Model file for the job. Use its own axes, mm. A direction names the side the tool comes from. Give positions to 0.01 mm unless a question says otherwise; leave off trailing zeros. Order: outer loops, then holes, each group sorted by start corner. A loop starts at its lowest first (then second) coordinate and runs counter-clockwise, first axis right, second up. Notation, with made-up numbers: (33, -26) -> (46, -26) arc R30 cw to (46, 7) -> close; hole circle Ø2 at (68, 55.25). An arc over 180 degrees is marked (long way). Use CSV: the item, a comma, the result in double quotes. Start each with the question number.
1. Cut at C-C on y = -6.25. List the corners of the cut face in (x, z), then the cut area to 3 significant figures.
2. Wall check: line 1 (Y direction, x = 0, z = 5.65); line 2 (X direction, y = 8, z = 11.5); line 3 (X direction, y = 1.5, z = 15.25). Give the ranges that are in metal, low to high. Write a range as from..to.
3. Cut at A-A on z = 10.5. List the corners of the cut face in (x, y), then the cut area to 3 significant figures.
4. Cut at D-D on x = 11.5. List the corners of the cut face in (y, z).
5. Drop flat-ended pins along their axis: pin 1 (2.5 mm diameter, centred on y = -7, z = 3, fed in from +X); pin 2 (1 mm diameter, centred on x = 5.5, y = -7, fed in from -Z); pin 3 (0.7 mm diameter, centred on y = 6, z = 3, fed in from -X). Give the stop position or say it passes through.
6. Cut at B-B on z = 3. List the corners of the cut face in (x, y).
7. 3-axis set-ups, long thin cutter, end or side, ignore diameter. For faces 1 (the flat face through (17.75, 0, 12)), 2 (the flat face through (12, 8, 5)), 3 (the cylindrical face through (0, 10, 2)): which of +Z, -Z, +X, -X, +Y, -Y reach the whole face in a straight line?
8. Pull direction Y, two halves, no side cores. Call faces 4 (the flat face through (15, 9.75, 12)), 5 (the cylindrical face through (0.55, 8.01, 5.99)), 6 (the flat face through (-3.95, -6, 2)): released by +Y, released by -Y, zero draft, split by the parting line, or undercut.
```python
from build123d import *

# Parameters (mm, degrees)
SALIENTE_EXTRUIR1_DEPTH = 5
CROQUIS2_W              = 40
CROQUIS2_H              = 23
SALIENTE_EXTRUIR2_DEPTH = 2
SALIENTE_EXTRUIR3_DEPTH = 10
CROQUIS4_R              = 0.75
CORTAR_EXTRUIR1_DEPTH   = 10


with BuildPart() as part:
    # Croquis1 → Saliente-Extruir1 (new body)
    with BuildSketch(Plane.XY):
        with BuildLine():
            Line((-3.95, -5.119042668), (-16.364400449, -3.983366957))
            ThreePointArc((-16.364400449, -3.983366957), (-20, 0), (-16.364400449, 3.983366957))
            Line((-16.364400449, 3.983366957), (-3.95, 5.119042668))
            Line((-3.95, 5.119042668), (-3.95, 7.55))
            ThreePointArc((-3.95, 7.55), (0, 11.5), (3.95, 7.55))
            Line((3.95, 7.55), (3.95, 5.119042668))
            Line((3.95, 5.119042668), (16.364400449, 3.983366957))
            ThreePointArc((16.364400449, 3.983366957), (20, 0), (16.364400449, -3.983366957))
            Line((16.364400449, -3.983366957), (3.95, -5.119042668))
            Line((3.95, -5.119042668), (3.95, -7.55))
            ThreePointArc((3.95, -7.55), (0, -11.5), (-3.95, -7.55))
            Line((-3.95, -7.55), (-3.95, -5.119042668))
        make_face()
        with BuildLine():
            Line((-2.45, 3.75), (-16.227750281, 2.489604348))
            ThreePointArc((-16.227750281, 2.489604348), (-18.5, 0), (-16.227750281, -2.489604348))
            Line((-16.227750281, -2.489604348), (-2.45, -3.75))
            Line((-2.45, -3.75), (-2.45, -7.55))
            ThreePointArc((-2.45, -7.55), (0, -10), (2.45, -7.55))
            Line((2.45, -7.55), (2.45, -3.75))
            Line((2.45, -3.75), (16.227750281, -2.489604348))
            ThreePointArc((16.227750281, -2.489604348), (18.5, 0), (16.227750281, 2.489604348))
            Line((16.227750281, 2.489604348), (2.45, 3.75))
            Line((2.45, 3.75), (2.45, 7.55))
            ThreePointArc((2.45, 7.55), (0, 10), (-2.45, 7.55))
            Line((-2.45, 7.55), (-2.45, 3.75))
        make_face(mode=Mode.SUBTRACT)
    extrude(amount=SALIENTE_EXTRUIR1_DEPTH)

    # Croquis2 → Saliente-Extruir2 (add)
    with BuildSketch(Plane.XY.offset(5)):
        Rectangle(CROQUIS2_W, CROQUIS2_H)
    extrude(amount=SALIENTE_EXTRUIR2_DEPTH)

    # Croquis3 → Saliente-Extruir3 (add)
    with BuildSketch(Plane.XY.offset(7)):
        Polygon((-10, 7.25), (-10, 9.75), (-20, 9.75), (-20, -9.75), (-10, -9.75), (-10, -7.25), (-17.75, -7.25), (-17.75, 7.25), align=None)
        Polygon((17.75, 7.25), (17.75, -7.25), (10, -7.25), (10, -9.75), (20, -9.75), (20, 9.75), (10, 9.75), (10, 7.25), align=None)
    extrude(amount=SALIENTE_EXTRUIR3_DEPTH)

    # Croquis4 → Cortar-Extruir1 (cut)
    with BuildSketch(Plane(origin=(0, 0, 5), x_dir=(-1, 0, 0), z_dir=(0, 0, -1))):
        with Locations((0, -7.5)):
            Circle(CROQUIS4_R)
        with Locations((0, 7.5)):
            Circle(CROQUIS4_R)
    extrude(amount=-CORTAR_EXTRUIR1_DEPTH, mode=Mode.SUBTRACT)


solid = part.part
```
Verdict:
1,outline,"(-20, 5) -> (-3.95, 5) -> (-3.95, 0) -> (-2.45, 0) -> (-2.45, 5) -> (2.45, 5) -> (2.45, 0) -> (3.95, 0) -> (3.95, 5) -> (20, 5) -> (20, 17) -> (17.75, 17) -> (17.75, 7) -> (-17.75, 7) -> (-17.75, 17) -> (-20, 17) -> close"
1,area,"140 mm^2"
2,line 1,"-11.5..-8.25, -6.75..6.75, 8.25..11.5"
2,line 2,"-20..-10, 10..20"
2,line 3,"-20..-17.75, 17.75..20"
3,outline,"(-20, -9.75) -> (-10, -9.75) -> (-10, -7.25) -> (-17.75, -7.25) -> (-17.75, 7.25) -> (-10, 7.25) -> (-10, 9.75) -> (-20, 9.75) -> close; (10, -9.75) -> (20, -9.75) -> (20, 9.75) -> (10, 9.75) -> (10, 7.25) -> (17.75, 7.25) -> (17.75, -7.25) -> (10, -7.25) -> close"
3,area,"165 mm^2"
4,outline,"(-11.5, 5) -> (-4.43, 5) -> (-4.43, 0) -> (-2.92, 0) -> (-2.92, 5) -> (2.92, 5) -> (2.92, 0) -> (4.43, 0) -> (4.43, 5) -> (11.5, 5) -> (11.5, 7) -> (9.75, 7) -> (9.75, 17) -> (7.25, 17) -> (7.25, 7) -> (-7.25, 7) -> (-7.25, 17) -> (-9.75, 17) -> (-9.75, 7) -> (-11.5, 7) -> close"
5,pin 1,"x = 3.95"
5,pin 2,"z = 5"
5,pin 3,"x = -3.95"
6,outline,"(-16.36, -3.98) -> (-3.95, -5.12) -> (-3.95, -7.55) arc R3.95 ccw to (3.95, -7.55) -> (3.95, -5.12) -> (16.36, -3.98) arc R4 ccw to (16.36, 3.98) -> (3.95, 5.12) -> (3.95, 7.55) arc R3.95 ccw to (-3.95, 7.55) -> (-3.95, 5.12) -> (-16.36, 3.98) arc R4 ccw to start; hole (-16.23, -2.49) -> (-2.45, -3.75) -> (-2.45, -7.55) arc R2.45 ccw to (2.45, -7.55) -> (2.45, -3.75) -> (16.23, -2.49) arc R2.5 ccw to (16.23, 2.49) -> (2.45, 3.75) -> (2.45, 7.55) arc R2.45 ccw to (-2.45, 7.55) -> (-2.45, 3.75) -> (-16.23, 2.49) arc R2.5 ccw to start"
7,face 1,"+Z"
7,face 2,"-Z, +X, +Y"
7,face 3,"-Z"
8,face 4,"released by +Y"
8,face 5,"undercut"
8,face 6,"zero draft"
